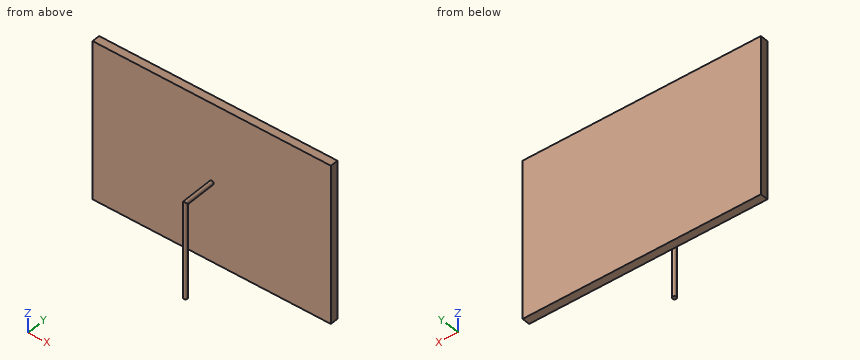
```python
from build123d import *

# Parameters (mm, degrees)
F0_W     = 762
F0_H     = 508
F1_DEPTH = 25.4
F3_R     = 6.35


with BuildPart() as f1:
    # F0 (on Front) → F1 (new body)
    with BuildSketch(Plane.XZ):
        Rectangle(F0_W, F0_H)
    extrude(amount=F1_DEPTH)

    # F4: sweep along a path in F2
    with BuildLine(Plane.YZ) as f4_path:
        Line((0, 0), (-127, 0))
        Line((-127, 0), (-127, -304.8))
    # F3 (on Front) → F4 (sweep)
    with BuildSketch(Plane.XZ):
        Circle(F3_R)
    sweep(path=f4_path.line, transition=Transition.RIGHT)


solid = f1.part
```
Here's how the part is built. I have some questions about the finished solid (model axes, mm). Round coordinates to 2 decimals unless told otherwise and drop trailing zeros. Write each loop counter-clockwise with the first axis right and the second up, starting at its lowest first coordinate (ties: lowest second). Pieces come first, ordered by that corner, then holes.
Q1. If we section it at C-C on x = 253: Write out the boundary of the cut face in (y, z).
Q2. Will these pins go through, and if not, where does the flat tip stop? P1, Ø6, axis at x = 82.5, z = -55.5, coming from the -Y side; P2, Ø10, axis at y = -111, z = -184.5, coming from the +X side; P3, Ø5, axis at x = -7.5, y = -94, coming from the +Z side; P4, Ø1.5, axis at x = 83.5, y = -23, coming from the -Z side.
Q3. Please list where these lines run through material, in increasing order: probe 1 along Y at (x, z) = (-173, -12); probe 2 along Z at (x, y) = (343, -10.5).
Q4. If we section it at B-B on y = -8.5: Write out the boundary of the cut face in (x, z), plus the area to 3 significant figures.
Q5. If we section it at A-A on z = -25: Write out the boundary of the cut face in (x, y), plus the area to 3 significant figures.
Q6. If we section it at D-D on y = -75: Write out the boundary of the cut face in (x, z), plus the area to 3 significant figures.
Answer below:
1. outline: (-25.4, -254) - (0, -254) - (0, 254) - (-25.4, 254) - close
2. P1: stops at y = -25.4
2. P2: passes through
2. P3: stops at z = 3.91
2. P4: stops at z = -254
3. probe 1: y = -25.4 to 0
3. probe 2: z = -254 to 254
4. outline: (-381, -254) - (381, -254) - (381, 254) - (-381, 254) - close
4. area: 387,000 mm2
5. outline: (-381, -25.4) - (381, -25.4) - (381, 0) - (-381, 0) - close; circle Ø12.7 at (0, -127)
5. area: 19,500 mm2
6. outline: circle Ø12.7 at (0, 0)
6. area: 127 mm2
